Source: CAD feature listing. Evaluate the final solid. Frame: model axes, mm. A direction names the side the tool comes from. Round coordinates to 2 decimals unless told otherwise and drop trailing zeros. Write each loop counter-clockwise with the first axis right and the second up, starting at its lowest first coordinate (ties: lowest second). Pieces come first, ordered by that corner, then holes. Notation, with made-up numbers: M 61.25,79.25 L 104.25,79.25 A19 ccw 104.25,102.25 Z; hole C -8.75,89 d5. An arc over 180 degrees is marked long. Answer in a Markdown table with one row per item. Add a question column.
Item 1: Cut plane B-B on x = 19. Return loops of the section in (y, z).
Item 2: Material intervals for probe 1 along Y at (x, z) = (-19, 1.65), sorted ascending.
Item 3: Mould query, pull axis X, two halves, no side actions, for faces 1 (the face through (17.62, -8.83, 1.45)), 2 (the face through (12, -9.208, 1)), 3 (the face through (6.096, -7, 1)). Classes: released by +X, released by -X, zero draft, split by the parting line, or undercut.
Item 4: Contact query for a flat-ended pin moving along its axis: pin 1 (1 mm diameter, centred on y = -7.5, z = 1, fed in from -X). Output: stop coordinate, or through.
Item 5: Set-up query: faces 4 (the face through (0, -1, 0)), 5 (the face through (0, -1, 2.858)), 6 (the face through (-18.288, -7, 1)), 7 (the face through (20, -6.35, 1)), 8 (the face through (-6.096, -7, 1)). Return all of +Z, -Z, +X, -X, +Y, -Y with unobstructed straight access to the full face (end or side cutting, diameter ignored); none if empty.
from build123d import *

# Parameters (mm, degrees)
SKETCH1_W             = 44.45
SKETCH1_H             = 12.7
BOSS_EXTRUDE1_DEPTH   = 2.8575
SKETCH2_W             = 12.192
SKETCH2_H             = 2.8575
BOSS_EXTRUDE2_DEPTH   = 2.8575
CHAMFER1_SIZE         = 0.762
CHAMFER1_SIZE2        = 1.319822715
CHAMFER1_PART_2_SIZE  = 0.762
CHAMFER1_PART_2_SIZE2 = 1.319822715
CHAMFER2_SIZE         = 0.762
CHAMFER2_SIZE2        = 1.319822715
CHAMFER2_PART_2_SIZE  = 0.762
CHAMFER2_PART_2_SIZE2 = 1.319822715


with BuildPart() as part:
    # Sketch1 → Boss-Extrude1 (new body)
    with BuildSketch(Plane.XY):
        Rectangle(SKETCH1_W, SKETCH1_H)
    extrude(amount=BOSS_EXTRUDE1_DEPTH)

    # Sketch2 → Boss-Extrude2 (add)
    with BuildSketch(Plane(origin=(0, -6.35, 0), x_dir=(-1, 0, 0), z_dir=(0, -1, 0))):
        with Locations((12.192, -1.42875)):
            Rectangle(SKETCH2_W, SKETCH2_H)
        with Locations((-12.192, -1.42875)):
            Rectangle(SKETCH2_W, SKETCH2_H)
    extrude(amount=BOSS_EXTRUDE2_DEPTH)

    # Chamfer1
    chamfer1_edges = [part.edges().sort_by_distance(p)[0] for p in [
        (-18.288, -9.2075, 1.42875),
    ]]
    chamfer1_side = [part.faces().sort_by_distance(p)[0] for p in [
        (-18.288, -7.77875, 1.42875),
    ]]
    chamfer(chamfer1_edges, length=CHAMFER1_SIZE, length2=CHAMFER1_SIZE2, reference=chamfer1_side[0])

    # Chamfer1 part 2
    chamfer1_part_2_edges = [part.edges().sort_by_distance(p)[0] for p in [
        (6.096, -9.2075, 1.42875),
    ]]
    chamfer1_part_2_side = [part.faces().sort_by_distance(p)[0] for p in [
        (6.096, -7.77875, 1.42875),
    ]]
    chamfer(chamfer1_part_2_edges, length=CHAMFER1_PART_2_SIZE, length2=CHAMFER1_PART_2_SIZE2, reference=chamfer1_part_2_side[0])

    # Chamfer2
    chamfer2_edges = [part.edges().sort_by_distance(p)[0] for p in [
        (-6.096, -9.2075, 1.42875),
    ]]
    chamfer2_side = [part.faces().sort_by_distance(p)[0] for p in [
        (-6.096, -7.77875, 1.42875),
    ]]
    chamfer(chamfer2_edges, length=CHAMFER2_SIZE, length2=CHAMFER2_SIZE2, reference=chamfer2_side[0])

    # Chamfer2 part 2
    chamfer2_part_2_edges = [part.edges().sort_by_distance(p)[0] for p in [
        (18.288, -9.2075, 1.42875),
    ]]
    chamfer2_part_2_side = [part.faces().sort_by_distance(p)[0] for p in [
        (18.288, -7.77875, 1.42875),
    ]]
    chamfer(chamfer2_part_2_edges, length=CHAMFER2_PART_2_SIZE, length2=CHAMFER2_PART_2_SIZE2, reference=chamfer2_part_2_side[0])


solid = part.part
Results below:
| question | item | result |
|---|---|---|
| 1 | outline | M -6.35,0 L 6.35,0 L 6.35,2.86 L -6.35,2.86 Z |
| 2 | probe 1 | -6.35 to 6.35 |
| 3 | face 1 | released by +X |
| 3 | face 2 | zero draft |
| 3 | face 3 | undercut |
| 4 | pin 1 | x = -18.29 |
| 5 | face 4 | -Z, +X, -X, +Y, -Y |
| 5 | face 5 | +Z, +X, -X, +Y, -Y |
| 5 | face 6 | +Z, -Z, -X, -Y |
| 5 | face 7 | +Z, -Z, +X, -Y |
| 5 | face 8 | +Z, -Z, -Y |
